Read the model definition and answer for the solid it produces. Units are mm, in the model's axes. A direction names the side the tool comes from. Round coordinates to 2 decimals unless told otherwise and drop trailing zeros. Write each loop counter-clockwise with the first axis right and the second up, starting at its lowest first coordinate (ties: lowest second). Pieces come first, ordered by that corner, then holes. Notation, with made-up numbers: (37.25, 53) -> (92.25, 53) arc R26 ccw to (92.25, 74) -> close; hole circle Ø7 at (6.5, 61). An arc over 180 degrees is marked (long way). Return JSON: item names as keys, results as strings. Group by question number.
(1) A cutting plane is placed at A-A on x = 19. Give the vertices of the cut face in (y, z).
(2) For faces 4 (the flat face through (19, 2, -27.239)), 5 (the cylindrical face through (-12.145, 2.028, 1.859)), determine the directions among +Z, -Z, +X, -X, +Y, -Y from which every point of the face is accessible in a straight line to the end or side of a thin tool.
(3) A cutting plane is placed at D-D on z = -5.5. Give the vertices of the cut face in (x, y), then the cut area to 3 significant figures.
(4) Straight lines are drawn through the part: line 1 (Z direction, x = 19, y = 1.85); line 2 (Z direction, x = -10, y = 1.5); line 3 (X direction, y = 3.45, z = -19.5). For each, find the intervals that lie inside material, in ascending order.
(5) The mould has two halves that part along X. Classify faces 1 (the cylindrical face through (-10.794, 2.028, -19.63)), 2 (the cylindrical face through (33.1, 1.97, -26.38)), 3 (the flat face through (10, 2, 2.761)): released by +X, released by -X, zero draft, split by the parting line, or undercut.
(6) A cutting plane is placed at B-B on z = -22. Give the vertices of the cut face in (x, y).
(7) Given pin 1 (1 mm diameter, centred on x = 22.5, y = 2, fed in from -Z), flat-ended and moving along its own axis, determine where the tip first touches the part or whether it passes through.
(8) A cutting plane is placed at C-C on x = 11. Give the vertices of the cut face in (y, z).
Autodesk Inventor part; units mm, degrees
ref_plane "YZ Plane" through (0, 0, 0) normal (1, 0, 0) x (0, 1, 0)
ref_plane "XZ Plane" through (0, 0, 0) normal (0, 1, 0) x (-1, 0, 0)
ref_plane "XY Plane" through (0, 0, 0) normal (0, 0, 1) x (1, 0, 0)
sketch "Sketch1" plane through (0, 0, 0) normal (0, 1, 0) x (-1, 0, 0)
  line L0 (13, 2.7611) -> (-25, 2.7611)
  line L1 (-25, 2.7611) -> (-25, -27.2389)
  line L2 (-25, -27.2389) -> (13, -27.2389)
  line L3 (13, -27.2389) -> (13, 2.7611)
  circle A0 centre (-10, -4.2389) radius 2.75
  line L4 (-4.8021, -1.4889) -> (-20.6552, -1.4889)
  line L5 (-20.6552, -1.4889) -> (-20.6552, -6.9889)
  line L6 (-20.6552, -6.9889) -> (-4.8021, -6.9889)
  line L7 (-4.8021, -6.9889) -> (-4.8021, -1.4889)
  circle A1 centre (-4.8021, -4.2389) radius 2.75
  circle A2 centre (-20.6552, -4.2389) radius 2.75
  point P0 (0, 0)
  point P1 (-20.6552, -1.4889)
  point P2 (-4.8021, -1.4889)
  point P3 (-10, -6.9889)
  point P4 (-10, -1.4889)
  dimension "d0" = 15
  dimension "d1" = 38
  dimension "d2" = 5.5
  dimension "d3" = 7
  dimension "d4" = 30
extrude "Extrusion1" add sketch "Sketch1" along normal blind 4 contours L3 L2 L1 L0 | A0 A1 L7 | A0 L4 A1 | A1 L6 A0 | A1 L7
sketch "Sketch2" plane through (0, 4, 0) normal (0, 1, 0) x (1, 0, 0)
  line L0 (-13, -2.7611) -> (25, -2.7611)
  line L1 (25, -2.7611) -> (34, -2.7611)
  line L2 (34, -2.7611) -> (34, 27.2389)
  line L3 (34, 27.2389) -> (25, 27.2389)
  line L4 (25, 27.2389) -> (25, -2.7611)
  line L5 (25, 27.2389) -> (-13, 27.2389)
  point P0 (0, 0)
  dimension "d11" = 9
extrude "Extrusion2" add sketch "Sketch2" against normal up to surface (4 mm away)
sketch "Sketch3" plane through (0, 4, 0) normal (0, 1, 0) x (1, 0, 0)
  circle A0 centre (20.6552, 20.2389) radius 2.75
  line L0 (34, 27.2389) -> (-13, 27.2389)
  arc A1 (20.6552, 1.4889) -> (20.6552, 6.9889) centre (20.6552, 4.2389) ccw
  circle A2 centre (10, 20.2389) radius 2.75
  line L1 (10, 17.4889) -> (20.6552, 17.4889)
  line L2 (20.6552, 17.4889) -> (20.6552, 22.9889)
  line L3 (20.6552, 22.9889) -> (10, 22.9889)
  line L4 (10, 22.9889) -> (10, 17.4889)
  point P0 (0, 0)
  point P1 (10, 22.9889)
  point P2 (20.6552, 17.4889)
  dimension "d15" = 5.5
  dimension "d14" = 7
extrude "Extrusion3" cut sketch "Sketch3" against normal blind 10
sketch "Sketch4" plane through (0, 4, 0) normal (0, 1, 0) x (1, 0, 0)
  line L0 (-13, 27.2389) -> (-13, -2.7611)
  line L1 (-13, 15.4131) -> (3, 15.4131)
  line L2 (3, 15.4131) -> (3, 32.2389)
  line L3 (3, 32.2389) -> (-13, 32.2389)
  line L4 (-13, 32.2389) -> (-13, 15.4131)
  line L5 (34, 27.2389) -> (-13, 27.2389)
  point P0 (0, 0)
  point P1 (-13, 27.2389)
  point P2 (3, 27.2389)
  dimension "d18" = 16
  dimension "d19" = 5
extrude "Extrusion4" add sketch "Sketch4" against normal up to surface (4 mm away) contours L4 L3 L2 L5
sketch "Sketch5" plane through (0, 4, 0) normal (0, 1, 0) x (1, 0, 0)
  circle A0 centre (-10, 29.2389) radius 1
  circle A1 centre (-10, 20.2389) radius 1
  line L0 (-13, 32.2389) -> (-13, -2.7611)
  line L1 (3, 32.2389) -> (-13, 32.2389)
  point P0 (0, 0)
  dimension "d22" = 2
  dimension "d23" = 9
  dimension "d24" = 3
  dimension "d25" = 3
extrude "Extrusion5" cut sketch "Sketch5" against normal through all
fillet "Fillet1" radius 3 6 edges at (3, 2, -27.2389) (3, 2, -32.2389) (-13, 2, -32.2389) (34, 2, -27.2389) (34, 2, 2.7611) (-13, 2, 2.7611)
sketch "Sketch7" plane through (0, 4, 0) normal (0, 1, 0) x (1, 0, 0)
  arc A0 (10, 6.9889) -> (10, 1.4889) centre (10, 4.2389) ccw
  line L0 (10, 6.9889) -> (20.6552, 6.9889)
  line L1 (20.6552, 1.4889) -> (10, 1.4889)
  arc A1 (20.6552, 1.4889) -> (20.6552, 6.9889) centre (20.6552, 4.2389) ccw
  line L2 (20.6552, 17.4889) -> (10, 17.4889)
  line L3 (10, 22.9889) -> (20.6552, 22.9889)
  arc A2 (10, 22.9889) -> (10, 17.4889) centre (10, 20.2389) ccw
  arc A3 (20.6552, 17.4889) -> (20.6552, 22.9889) centre (20.6552, 20.2389) ccw
  circle A4 centre (19, 4.2389) radius 2.5
  circle A5 centre (19, 20.2389) radius 2.5
  line L4 (34, 0.2389) -> (34, 24.2389)
  point P0 (0, 0)
  dimension "d31" = 5
  dimension "d32" = 15
extrude "Extrusion7" add sketch "Sketch7" against normal up to surface (4 mm away)
properties part number "ystop"
Checks:
{
 "1": {"outline": "(0, -27.24) -> (4, -27.24) -> (4, -22.74) -> (0, -22.74) -> close; (0, -17.74) -> (4, -17.74) -> (4, -6.74) -> (0, -6.74) -> close; (0, -1.74) -> (4, -1.74) -> (4, 2.76) -> (0, 2.76) -> close"},
 "2": {"face 4": "-Z, +X, +Y, -Y", "face 5": "+Z, -X, +Y, -Y"},
 "3": {"outline": "(-13, 0) -> (16.84, 0) -> (16.84, 4) -> (-13, 4) -> close; (21.16, 0) -> (34, 0) -> (34, 4) -> (21.16, 4) -> close", "area": "171 mm^2"},
 "4": {"line 1": "z = -27.24 to -22.74, -17.74 to -6.74, -1.74 to 2.76", "line 2": "z = -32.24 to -30.24, -28.24 to -21.24, -19.24 to 2.76", "line 3": "x = -13 to -10.67, -9.33 to 16.61, 21.39 to 34"},
 "5": {"face 1": "undercut", "face 2": "released by +X", "face 3": "zero draft"},
 "6": {"outline": "(-13, 0) -> (17.23, 0) -> (17.23, 4) -> (-13, 4) -> close; (20.77, 0) -> (34, 0) -> (34, 4) -> (20.77, 4) -> close"},
 "7": {"pin 1": "stops at z = -27.24"},
 "8": {"outline": "(0, -27.24) -> (4, -27.24) -> (4, 2.76) -> (0, 2.76) -> close"}
}
